from build123d import *

# Parameters (mm, degrees)
F0_W     = 30
F0_H     = 30
F1_DEPTH = 40
F3_D     = 12
F5_D     = 5.5
F6_R     = 5
F7_R     = 2


with BuildPart() as f1:
    # F0 (on Front) → F1 (new body)
    with BuildSketch(Plane.XZ):
        with Locations((15, 15)):
            Rectangle(F0_W, F0_H)
    extrude(amount=F1_DEPTH)

    # F3 (through all)
    with Locations(Plane.XY.offset(30)):
        with Locations((15, -20)):
            Hole(F3_D / 2)

    # F5 (through all)
    with Locations(Plane.YZ.offset(30)):
        with Locations((-30, 25), (-10, 25), (-10, 5), (-30, 5)):
            Hole(F5_D / 2)

    # F6
    f6_edges = [f1.edges().sort_by_distance(p)[0] for p in [
        (30, 0, 15),
        (30, -40, 15),
    ]]
    fillet(f6_edges, radius=F6_R)

    # F7
    f7_edges = [f1.edges().sort_by_distance(p)[0] for p in [
        (30, -20, 30),
        (30, -20, 0),
    ]]
    fillet(f7_edges, radius=F7_R)


solid = f1.part
The listing builds one solid part. Answer for the finished solid, in the listing's coordinates (mm). Coordinates: 2 decimals unless noted, no trailing zeros. Order: outer loops, then holes, each group sorted by start corner. A loop starts at its lowest first (then second) coordinate and runs counter-clockwise, first axis right, second up. Notation, with made-up numbers: (-5.5, 77.5) -> (51.5, 77.5) arc R14 cw to (51.5, 96.5) -> close; hole circle Ø3 at (46.5, 14). An arc over 180 degrees is marked (long way). Answer in a Markdown table with one row per item. Add a question column.
Item 1: Find section C-C (y = -20). Write down the section's boundary in (x, z).
Item 2: Find section D-D (y = -10). Write down the section's boundary in (x, z), then the cut area to 3 significant figures.
Item 3: Determine the mould class of faces 1 (the face through (12.32, -39.4, 0.57)), 2 (the face through (29.43, -20.21, 29.4)), 3 (the face through (14.79, -27.253, 5.121)) for opening direction Y: +Y half, -Y half, draft (parallel to the pull), parting line (faces both ways), or undercut.
Item 4: Find section B-B (z = 5). Write down the section's boundary in (x, y), then the cut area to 3 significant figures.
Item 5: Find section A-A (x = 15). Write down the section's boundary in (y, z), then the cut area to 3 significant figures.
Item 6: Find the intervals of material crossed by L1, parallel to Z at x = 20.5, y = -10; L2, parallel to Y at x = 5.25, z = 24.75; L3, parallel to Z at x = 24.5, y = -11, in increasing order. Write a range as from..to.
Result set:
| question | item | result |
|---|---|---|
| 1 | outline | (0, 0) -> (9, 0) -> (9, 30) -> (0, 30) -> close; (21, 0) -> (28, 0) arc R2 ccw to (30, 2) -> (30, 28) arc R2 ccw to (28, 30) -> (21, 30) -> close |
| 2 | outline | (0, 0) -> (28, 0) arc R2 ccw to (30, 2) -> (30, 2.25) -> (0, 2.25) -> close; (0, 7.75) -> (30, 7.75) -> (30, 22.25) -> (0, 22.25) -> close; (0, 27.75) -> (30, 27.75) -> (30, 28) arc R2 ccw to (28, 30) -> (0, 30) -> close |
| 2 | area | 568 mm² |
| 3 | face 1 | -Y half |
| 3 | face 2 | draft |
| 3 | face 3 | undercut |
| 4 | outline | (0, -40) -> (25, -40) arc R5 ccw to (30, -35) -> (30, -32.75) -> (0, -32.75) -> close; (0, -27.25) -> (30, -27.25) -> (30, -12.75) -> (0, -12.75) -> close; (0, -7.25) -> (30, -7.25) -> (30, -5) arc R5 ccw to (25, 0) -> (0, 0) -> close; hole circle Ø12 at (15, -20) |
| 4 | area | 746 mm² |
| 5 | outline | (-40, 2) arc R2 ccw to (-38, 0) -> (-26, 0) -> (-26, 30) -> (-38, 30) arc R2 ccw to (-40, 28) -> close; (-14, 0) -> (-2, 0) arc R2 ccw to (0, 2) -> (0, 28) arc R2 ccw to (-2, 30) -> (-14, 30) -> close; hole circle Ø5.5 at (-30, 5); hole circle Ø5.5 at (-30, 25); hole circle Ø5.5 at (-10, 5); hole circle Ø5.5 at (-10, 25) |
| 5 | area | 742 mm² |
| 6 | L1 | z = 0..2.25, 7.75..22.25, 27.75..30 |
| 6 | L2 | y = -40..-32.74, -27.26..-12.74, -7.26..0 |
| 6 | L3 | z = 0..2.44, 7.56..22.44, 27.56..30 |
